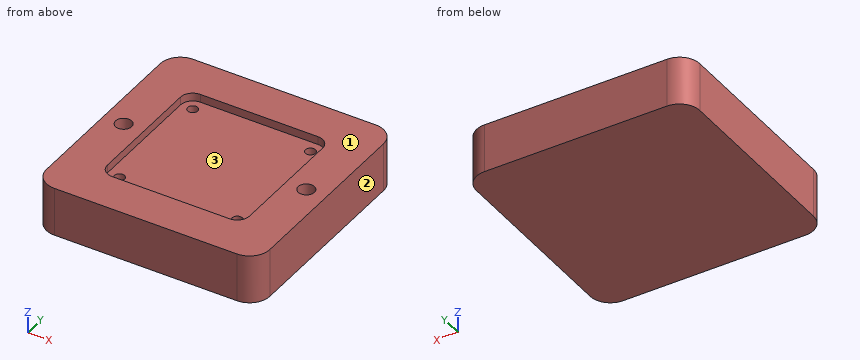
```python
from build123d import *

# Parameters (mm, degrees)
BOSS_EXTRUDE1_DEPTH             = 4
BOSS_EXTRUDE2_DEPTH             = 20
F_8_0MM_DOWEL_HOLE1_D           = 8
F_8_0MM_DOWEL_HOLE1_DEPTH       = 18
F_8_0MM_DOWEL_HOLE1_TIP         = 2.403442476
TAP_DRILL_FOR_M6X1_0_TAP1_D     = 5
TAP_DRILL_FOR_M6X1_0_TAP1_DEPTH = 10
TAP_DRILL_FOR_M6X1_0_TAP1_TIP   = 1.502151548


with BuildPart() as part:
    # Sketch1 → Boss-Extrude1 (new body)
    with BuildSketch(Plane.XY):
        with BuildLine():
            Line((-45, 55), (45, 55))
            ThreePointArc((45, 55), (52.071067812, 52.071067812), (55, 45))
            Line((55, 45), (55, -45))
            ThreePointArc((55, -45), (52.071067812, -52.071067812), (45, -55))
            Line((45, -55), (-45, -55))
            ThreePointArc((-45, -55), (-52.071067812, -52.071067812), (-55, -45))
            Line((-55, -45), (-55, 45))
            ThreePointArc((-55, 45), (-52.071067812, 52.071067812), (-45, 55))
        make_face()
        with BuildLine():
            Line((-29, 35), (29, 35))
            ThreePointArc((29, 35), (33.242640687, 33.242640687), (35, 29))
            Line((35, 29), (35, -29))
            ThreePointArc((35, -29), (33.242640687, -33.242640687), (29, -35))
            Line((29, -35), (-29, -35))
            ThreePointArc((-29, -35), (-33.242640687, -33.242640687), (-35, -29))
            Line((-35, -29), (-35, 29))
            ThreePointArc((-35, 29), (-33.242640687, 33.242640687), (-29, 35))
        make_face(mode=Mode.SUBTRACT)
    extrude(amount=-BOSS_EXTRUDE1_DEPTH)

    # Sketch2 → Boss-Extrude2 (add)
    with BuildSketch(Plane.XY.offset(-4)):
        with BuildLine():
            Line((-45, -55), (45, -55))
            ThreePointArc((45, -55), (52.071067812, -52.071067812), (55, -45))
            Line((55, -45), (55, 45))
            ThreePointArc((55, 45), (52.071067812, 52.071067812), (45, 55))
            Line((45, 55), (-45, 55))
            ThreePointArc((-45, 55), (-52.071067812, 52.071067812), (-55, 45))
            Line((-55, 45), (-55, -45))
            ThreePointArc((-55, -45), (-52.071067812, -52.071067812), (-45, -55))
        make_face()
    extrude(amount=-BOSS_EXTRUDE2_DEPTH)

    # Ø8.0mm Dowel Hole1
    with Locations(Plane.XY):
        with Locations((-45, 0), (45, 0)):
            Hole(F_8_0MM_DOWEL_HOLE1_D / 2, depth=F_8_0MM_DOWEL_HOLE1_DEPTH)
            with Locations((0, 0, -(F_8_0MM_DOWEL_HOLE1_DEPTH + F_8_0MM_DOWEL_HOLE1_TIP / 2))):  # 118° drill point
                Cone(0, F_8_0MM_DOWEL_HOLE1_D / 2, F_8_0MM_DOWEL_HOLE1_TIP, mode=Mode.SUBTRACT)

    # Tap Drill for M6x1.0 Tap1
    with Locations(Plane.XY.offset(-4)):
        with Locations((-29, 29), (29, 29), (29, -29), (-29, -29)):
            Hole(TAP_DRILL_FOR_M6X1_0_TAP1_D / 2, depth=TAP_DRILL_FOR_M6X1_0_TAP1_DEPTH)
            with Locations((0, 0, -(TAP_DRILL_FOR_M6X1_0_TAP1_DEPTH + TAP_DRILL_FOR_M6X1_0_TAP1_TIP / 2))):  # 118° drill point
                Cone(0, TAP_DRILL_FOR_M6X1_0_TAP1_D / 2, TAP_DRILL_FOR_M6X1_0_TAP1_TIP, mode=Mode.SUBTRACT)


solid = part.part
```
Here's how the part is built. I have some questions about the finished solid (model axes, mm). Face numbers are marked on the shaded views. Coordinates: 2 decimals unless noted, no trailing zeros. Order: outer loops, then holes, each group sorted by start corner. A loop starts at its lowest first (then second) coordinate and runs counter-clockwise, first axis right, second up. Notation, with made-up numbers: (18, 2.5) - (29, 2.5) arc R18 cw to (29, 19.5) - close; hole circle Ø1 at (-16.75, 51). An arc over 180 degrees is marked (long way). One line per question, with ' | ' between items.
(1) Suppose I cut it at A-A on z = -12.25. List the corners of the cut face in (x, y) for me.
Report:
outline: (-55, -45) arc R10 ccw to (-45, -55) - (45, -55) arc R10 ccw to (55, -45) - (55, 45) arc R10 ccw to (45, 55) - (-45, 55) arc R10 ccw to (-55, 45) - close; hole circle Ø8 at (-45, 0); hole circle Ø5 at (-29, -29); hole circle Ø5 at (-29, 29); hole circle Ø5 at (29, -29); hole circle Ø5 at (29, 29); hole circle Ø8 at (45, 0)
(2) If we mould it in two halves opening along X, with no side actions, what happens to the marked faces 1, 2 and 3? For each: pulls with the +X half, pulls with the -X half, needs draft (parallel to the pull), parting line crosses it, or undercut.
Report:
face 1: needs draft | face 2: pulls with the +X half | face 3: undercut
(3) Will these pins go through, and if not, where does the flat tip stop? pin 1 (21 mm diameter, centred on x = 3, y = -5, fed in from +Z); pin 2 (4 mm diameter, centred on x = 29, y = 29, fed in from +Z).
Report:
pin 1: stops at z = -4 | pin 2: stops at z = -14.3
(4) If I drill on L1, parallel to X at y = 29, z = -9.25; L2, parallel to X at y = 0, z = -14.25, over which ranges is the centre line in solid material (lowest first)?
Report:
L1: x = -55 to -31.5, -26.5 to 26.5, 31.5 to 55 | L2: x = -55 to -49, -41 to 41, 49 to 55
(5) Suppose I cut it at B-B on y = -19.5. List the corners of the cut face in (x, z) for me, and give its area (3 significant figures).
Report:
outline: (-55, -24) - (55, -24) - (55, 0) - (35, 0) - (35, -4) - (-35, -4) - (-35, 0) - (-55, 0) - close | area: 2,360 mm2
